Here's how the part is built. I have some questions about the finished solid (model axes, mm). A direction names the side the tool comes from. Round coordinates to 2 decimals unless told otherwise and drop trailing zeros. Write each loop counter-clockwise with the first axis right and the second up, starting at its lowest first coordinate (ties: lowest second). Pieces come first, ordered by that corner, then holes. Notation, with made-up numbers: (32, 31.5) - (57, 31.5) arc R28 ccw to (57, 69.5) - close; hole circle Ø5 at (-16, -13.75). An arc over 180 degrees is marked (long way). Use one line per item in the form item = value. Start each with the question number.
1. Will these pins go through, and if not, where does the flat tip stop? pin 1 (2 mm diameter, centred on y = 3.5, z = 16, fed in from -X); pin 2 (4 mm diameter, centred on x = -5, z = 41, fed in from -Y); pin 3 (5 mm diameter, centred on y = -2.5, z = 82, fed in from -X).
2. Which directions (+Z, -Z, +X, -X, +Y, -Y) give clear straight access to the entire face, cutting with the end or side of a thin tool? Please do faces 1 (the cylindrical face through (-9.139, -14.334, 38.532)), 2 (the cylindrical face through (2.17, 9.76, 113.73)).
3. If I drill on line 1 along X through (y, z) = (-8, 88.5); line 2 along Z through (x, y) = (1, -11.5); line 3 along Y through (x, z) = (13, 45), over which ranges is the centre line in solid material (lowest first)?
4. I want a section at D-D, the plane z = 102.5. List the corners of the cut face in (x, y) for me.
5. I want a section at A-A, the plane y = 0. List the corners of the cut face in (x, z) for me.
6. I want a section at C-C, the plane z = 11. List the corners of the cut face in (x, y) for me, plus the area to 3 significant figures.
```python
from build123d import *


with BuildPart() as part:
    # Sketch → Revolution (revolve)
    with BuildSketch(Plane.XZ):
        Polygon((0, 0), (-17, 0), (-17, 76), (-13.5, 79.08), (-13.5, 95.08), (-10, 97), (-10, 130), (0, 130), align=None)
    revolve(axis=Axis((0, 0, 0), (0, 0, 1)))


solid = part.part
```
Model answer:
q1.pin_1 = -16.82
q1.pin_2 = -16.73
q1.pin_3 = -13.5
q2.face_1 = +Z, -Z
q2.face_2 = +Z
q3.line_1 = -10.87 to 10.87
q3.line_2 = 0 to 96.15
q3.line_3 = -10.95 to 10.95
q4.outline = circle Ø20 at (0, 0)
q5.outline = (-17, 0) - (17, 0) - (17, 76) - (13.5, 79.08) - (13.5, 95.08) - (10, 97) - (10, 130) - (-10, 130) - (-10, 97) - (-13.5, 95.08) - (-13.5, 79.08) - (-17, 76) - close
q6.outline = circle Ø34 at (0, 0)
q6.area = 908 mm2
